Source: CAD feature listing. Evaluate the final solid. Frame: model axes, mm. Give positions to 0.01 mm unless a question says otherwise; leave off trailing zeros. Write each loop counter-clockwise with the first axis right and the second up, starting at its lowest first coordinate (ties: lowest second). Pieces come first, ordered by that corner, then holes.
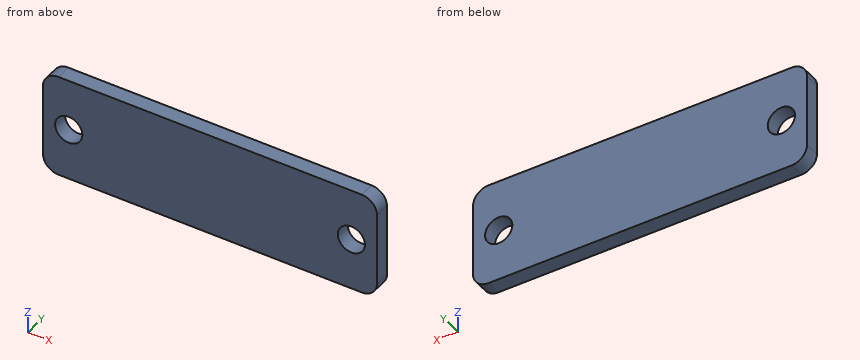
```python
from build123d import *

# Parameters (mm, degrees)
BOSS_EXTRUDE1_DEPTH  = 3
M3_CLEARANCE_HOLE1_D = 3.2
M5_CLEARANCE_HOLE1_D = 5.3
SKETCH8_W            = 65
SKETCH8_H            = 21.5
CUT_EXTRUDE1_DEPTH   = 4
FILLET2_R            = 3


with BuildPart() as part:
    # Sketch1 → Boss-Extrude1 (new body)
    with BuildSketch(Plane(origin=(0, 0, 0), x_dir=(1, 0, 0), z_dir=(0, 1, 0))):
        with BuildLine():
            Line((32.5, -29), (32.5, -9))
            Line((32.5, -9), (7.563621408, 9.951966197))
            ThreePointArc((7.563621408, 9.951966197), (0, 12.5), (-7.563621408, 9.951966197))
            Line((-7.563621408, 9.951966197), (-32.5, -9))
            Line((-32.5, -9), (-32.5, -29))
            Line((-32.5, -29), (32.5, -29))
        make_face()
        with BuildLine():
            ThreePointArc((-4, 0), (0, 4), (4, 0))
            ThreePointArc((4, 0), (0, -4), (-4, 0))
        make_face(mode=Mode.SUBTRACT)
    extrude(amount=BOSS_EXTRUDE1_DEPTH)

    # M3 Clearance Hole1 (through all)
    with Locations(Plane(origin=(0, 0, 0), x_dir=(-1, 0, 0), z_dir=(0, -1, 0))):
        with Locations((8.5, 0), (-8.5, 0)):
            Hole(M3_CLEARANCE_HOLE1_D / 2)

    # M5 Clearance Hole1 (through all)
    with Locations(Plane(origin=(0, 0, 0), x_dir=(-1, 0, 0), z_dir=(0, -1, 0))):
        with Locations((-27.5, -19), (27.5, -19)):
            Hole(M5_CLEARANCE_HOLE1_D / 2)

    # Sketch8 → Cut-Extrude1 (cut, through all)
    with BuildSketch(Plane(origin=(0, 0, 0), x_dir=(1, 0, 0), z_dir=(0, 1, 0))):
        with Locations((0, 1.75)):
            Rectangle(SKETCH8_W, SKETCH8_H)
    extrude(amount=CUT_EXTRUDE1_DEPTH, mode=Mode.SUBTRACT)

    # Fillet2
    fillet2_edges = [part.edges().sort_by_distance(p)[0] for p in [
        (32.5, 1.5, 9),
        (32.5, 1.5, 29),
        (-32.5, 1.5, 29),
        (-32.5, 1.5, 9),
    ]]
    fillet(fillet2_edges, radius=FILLET2_R)


solid = part.part
```
1. Section query C-C (y = 0.6). Return loops of the section in (x, z), plus the area to 3 significant figures.
2. Section query D-D (x = 27). Return loops of the section in (y, z), plus the area to 3 significant figures.
3. Section query B-B (z = 19). Return loops of the section in (x, y), plus the area to 3 significant figures.
4. Section query A-A (x = -27.5). Return loops of the section in (y, z).
5. Line query: probe 1 along X at (y, z) = (1.35, 19); probe 2 along Z at (x, y) = (-27.5, 0.6); probe 3 along X at (y, z) = (0.65, 19.75). Output: solid intervals per line, ascending.
The answers:
1. outline: (-32.5, 12) arc R3 ccw to (-29.5, 9) - (29.5, 9) arc R3 ccw to (32.5, 12) - (32.5, 26) arc R3 ccw to (29.5, 29) - (-29.5, 29) arc R3 ccw to (-32.5, 26) - close; hole circle Ø5.3 at (-27.5, 19); hole circle Ø5.3 at (27.5, 19)
1. area: 1,250 mm2
2. outline: (0, 9) - (3, 9) - (3, 16.4) - (0, 16.4) - close; (0, 21.6) - (3, 21.6) - (3, 29) - (0, 29) - close
2. area: 44.4 mm2
3. outline: (-32.5, 0) - (-30.15, 0) - (-30.15, 3) - (-32.5, 3) - close; (-24.85, 0) - (24.85, 0) - (24.85, 3) - (-24.85, 3) - close; (30.15, 0) - (32.5, 0) - (32.5, 3) - (30.15, 3) - close
3. area: 163 mm2
4. outline: (0, 9) - (3, 9) - (3, 16.35) - (0, 16.35) - close; (0, 21.65) - (3, 21.65) - (3, 29) - (0, 29) - close
5. probe 1: x = -32.5 to -30.15, -24.85 to 24.85, 30.15 to 32.5
5. probe 2: z = 9 to 16.35, 21.65 to 29
5. probe 3: x = -32.5 to -30.04, -24.96 to 24.96, 30.04 to 32.5
